from build123d import *

# Parameters (mm, degrees)
CROQUIS1_R              = 1.5
SALIENTE_EXTRUIR1_DEPTH = 10
SALIENTE_EXTRUIR2_DEPTH = 15
MATRIZL1_COUNT          = 2
MATRIZL1_PITCH          = 37.68964915
SALIENTE_EXTRUIR3_DEPTH = 13
SALIENTE_EXTRUIR7_DEPTH = 5
REDONDEO2_R             = 10
CROQUIS11_R             = 1.5
CORTAR_EXTRUIR2_DEPTH   = 5


with BuildPart() as part:
    # Croquis1 → Saliente-Extruir1 (new body)
    with BuildSketch(Plane(origin=(0, 0, 0), x_dir=(1, 0, 0), z_dir=(0, 1, 0))):
        Polygon((-189.195504205, 26.344824576), (-153.149960772, 26.344824576), (-153.149960772, 29.769862991), (-126.147833027, 29.769862991), (-126.147833027, -29.769862991), (-153.149960772, -29.769862991), (-153.149960772, -26.344824576), (-189.195504205, -26.344824576), align=None)
        with Locations(Location((-137.631197841, 26.344824576, 0), (0, 0, 270))):
            Circle(CROQUIS1_R, mode=Mode.SUBTRACT)
        with Locations(Location((-137.631197841, -26.344824576, 0), (0, 0, 90))):
            Circle(CROQUIS1_R, mode=Mode.SUBTRACT)
    extrude(amount=SALIENTE_EXTRUIR1_DEPTH)

    # Croquis3 → Saliente-Extruir2 (add)
    with BuildSketch(Plane.XY.offset(26.344824576)):
        Polygon((-189.195504205, 0), (-201.604805992, 12.545329197), (-220.943628409, 69.680078214), (-231.495067756, 78.724169083), (-209.43357333, 78.724169083), (-189.195504205, 18.932679451), (-166.427858451, 10), (-166.427858451, 0), align=None)
    saliente_extruir2 = extrude(amount=-SALIENTE_EXTRUIR2_DEPTH)

    # MatrizL1: Saliente-Extruir2 ×2
    with Locations(*[(0, 0, -i * MATRIZL1_PITCH) for i in range(1, MATRIZL1_COUNT)]):
        add(saliente_extruir2)

    # Croquis8 → Saliente-Extruir3 (add)
    with BuildSketch(Plane(origin=(-163.998418841, -55.509761627, 0), x_dir=(0, 0, -1), z_dir=(0.9472114013741786, 0.3206096709501519, 0))):
        Polygon((-11.344824576, 110.153008866), (-11.344824576, 104.748047896), (-3.12328674, 111.657611587), (-3.12328674, 63.690909236), (3.123286737, 63.690909236), (3.123286737, 111.657611587), (11.344824574, 104.748047896), (11.344824574, 110.153008866), (-1e-09, 119.687452364), align=None)
    extrude(amount=-SALIENTE_EXTRUIR3_DEPTH)

    # Croquis10 → Saliente-Extruir7 (add)
    with BuildSketch(Plane(origin=(0, 78.724169083, 0), x_dir=(1, 0, 0), z_dir=(0, 1, 0))):
        with BuildLine():
            Line((-214.43357333, 26.344824574), (-220.943628409, 26.344824574))
            Line((-220.943628409, 26.344824574), (-231.495067756, 39.001543724))
            Line((-231.495067756, 39.001543724), (-248.853619127, 39.65983126))
            Line((-248.853619127, 39.65983126), (-259.380857056, 25.173184149))
            Line((-259.380857056, 25.173184149), (-248.853619127, 10.686537038))
            Line((-248.853619127, 10.686537038), (-231.495067756, 11.344824574))
            Line((-231.495067756, 11.344824574), (-229.458019065, 3.999750012))
            Line((-229.458019065, 3.999750012), (-229.458019065, -4.057622202))
            Line((-229.458019065, -4.057622202), (-231.495067756, -11.402696763))
            Line((-231.495067756, -11.402696763), (-248.853619127, -10.744409227))
            Line((-248.853619127, -10.744409227), (-259.380857056, -25.231056338))
            Line((-259.380857056, -25.231056338), (-248.853619127, -39.71770345))
            Line((-248.853619127, -39.71770345), (-231.495067756, -39.059415914))
            Line((-231.495067756, -39.059415914), (-220.943628409, -26.402696763))
            Line((-220.943628409, -26.402696763), (-214.43357333, -26.402696763))
            ThreePointArc((-214.43357333, -26.402696763), (-210.898039424, -24.938230669), (-209.43357333, -21.402696763))
            Line((-209.43357333, -21.402696763), (-209.43357333, -16.36524325))
            Line((-209.43357333, -16.36524325), (-219.208523363, -1.818697081))
            Line((-219.208523363, -1.818697081), (-219.208523363, 1.760824892))
            Line((-219.208523363, 1.760824892), (-209.43357333, 16.30737106))
            Line((-209.43357333, 16.30737106), (-209.43357333, 21.344824574))
            ThreePointArc((-209.43357333, 21.344824574), (-210.898039424, 24.880358479), (-214.43357333, 26.344824574))
        make_face()
    extrude(amount=SALIENTE_EXTRUIR7_DEPTH)

    # Redondeo2
    # the kernel refuses this fillet: 10 mm, written as the material it takes off along each edge
    with BuildSketch(Plane(origin=(-196.732088511, 0.651068043, 27.595787298), x_dir=(-0.3206096709501526, 0.9472114013741784, 0), z_dir=(0, 0, -1))) as redondeo2_piece_1_section:
        with BuildLine():
            CenterArc((9.789000223, 10), REDONDEO2_R, 191.790853222, 78.209146778)
            Line((0, 7.956602185), (0, 0))
            Line((0, 0), (9.789000223, 0))
        make_face()
    redondeo2_piece_1 = extrude(amount=30.719074034, mode=Mode.PRIVATE)
    redondeo2_piece_1 = split(redondeo2_piece_1, bisect_by=Plane(origin=(-197.071889221, 5.655111801, 11.344824576), z_dir=(0, 0, -1)), keep=Keep.TOP, mode=Mode.PRIVATE)
    add(redondeo2_piece_1, mode=Mode.SUBTRACT)

    # Croquis11 → Cortar-Extruir2 (cut)
    with BuildSketch(Plane(origin=(0, 83.724169083, 0), x_dir=(1, 0, 0), z_dir=(0, 1, 0))):
        with Locations(Location((-241.678058983, 25.173184149, 0), (0, 0, 270))):
            Circle(CROQUIS11_R)
        with Locations(Location((-241.678058983, -25.173184149, 0), (0, 0, 90))):
            Circle(CROQUIS11_R)
    extrude(amount=-CORTAR_EXTRUIR2_DEPTH, mode=Mode.SUBTRACT)


solid = part.part
Verification items for the finished model (mm, model axes). A direction names the side the tool comes from. Coordinates: 2 decimals unless noted, no trailing zeros. Write each loop counter-clockwise with the first axis right and the second up, starting at its lowest first coordinate (ties: lowest second). Pieces come first, ordered by that corner, then holes. Notation, with made-up numbers: (61.25, -18.5) -> (98.25, -18.5) arc R6 cw to (98.25, -11.5) -> close; hole circle Ø11 at (89.5, 11). An arc over 180 degrees is marked (long way). One line per item, written item: value. Start each with the question number.
Q1. Cross-section at B-B on y = 15. Enter the section's corners in (x, z), and give its area (3 significant figures).
Q2. Access from +Z, -Z, +X, -X, +Y, -Y to the whole of each face (thin tool, end or side, straight path). Record for faces 4 (the flat face through (-210, 78.724, 25)), 5 (the cylindrical face through (-139.096, 4.93, -26.67)), 6 (the flat face through (-214.39, 81.19, -8.93)), 7 (the flat face through (-204.78, 44.97, -7.18)).
Q3. Go/stop test with flat-tipped pins: P1, Ø11, axis at x = -137, y = 4.5, coming from the -Z side; P2, Ø13, axis at x = -204, y = 32, coming from the -Z side; P3, Ø1.5, axis at y = 82.5, z = -19, coming from the +X side. Record where each tip stops, or that it passes through.
Q4. Mould release check, pull along X, two halves, no side actions. Record for faces 1 (the flat face through (-209.434, 81, 19)), 2 (the flat face through (-240.3, 81.19, -11.01)), 3 (the flat face through (-157, 0, 0)): pulls with the +X half, pulls with the -X half, needs draft (parallel to the pull), parting line crosses it, or undercut.
Q5. Cross-section at D-D on z = -18.5. Enter the section's corners in (x, y).
Q6. Thickness scan on L1, parallel to Y at x = -137, z = -24.5; L2, parallel to Y at x = -222.5, z = -7; L3, parallel to X at y = 57, z = -21. Record the ranges inside material, lowest first. Write a range as from..to.
Q7. Cross-section at A-A on y = 76. Enter the section's corners in (x, z).
Q8. Cross-section at C-C on x = -226.5. Enter the section's corners in (y, z).
Checked values:
1. outline: (-202.44, -26.34) -> (-179.17, -26.34) -> (-179.17, -11.34) -> (-202.44, -11.34) -> close; (-202.44, 11.34) -> (-179.17, 11.34) -> (-179.17, 26.34) -> (-202.44, 26.34) -> close; (-201.59, -3.12) -> (-187.86, -3.12) -> (-187.86, 3.12) -> (-201.59, 3.12) -> close
1. area: 784 mm²
2. face 4: +Z, +X, +Y
2. face 5: +Y, -Y
2. face 6: +X, +Y
2. face 7: +X, -Y
3. P1: stops at z = -29.77
3. P2: stops at z = -26.34
3. P3: stops at x = -209.43
4. face 1: pulls with the +X half
4. face 2: undercut
4. face 3: needs draft
5. outline: (-254.53, 78.72) -> (-231.5, 78.72) -> (-220.94, 69.68) -> (-201.6, 12.55) -> (-189.2, 0) -> (-126.15, 0) -> (-126.15, 10) -> (-166.43, 10) -> (-189.2, 18.93) -> (-209.43, 78.72) -> (-209.43, 83.72) -> (-254.53, 83.72) -> close
6. L1: y = 0..10
6. L2: y = 78.72..83.72
6. L3: x = -216.65..-202.08
7. outline: (-228.32, -26.34) -> (-208.51, -26.34) -> (-208.51, -11.34) -> (-228.32, -11.34) -> close; (-228.32, 11.34) -> (-208.51, 11.34) -> (-208.51, 26.34) -> (-228.32, 26.34) -> close
8. outline: (74.44, -26.34) -> (78.72, -26.34) -> (78.72, -33.01) -> (83.72, -33.01) -> (83.72, 33.07) -> (78.72, 33.07) -> (78.72, 26.34) -> (74.44, 26.34) -> (74.44, 11.34) -> (78.72, 11.34) -> (78.72, -11.34) -> (74.44, -11.34) -> close
